The listing builds one solid part. Answer for the finished solid, in the listing's coordinates (mm). A direction names the side the tool comes from. Give positions to 0.01 mm unless a question says otherwise; leave off trailing zeros. Write each loop counter-clockwise with the first axis right and the second up, starting at its lowest first coordinate (ties: lowest second). Pieces come first, ordered by that corner, then holes. Notation, with made-up numbers: (80.5, 17.5) - (86.5, 17.5) arc R19 ccw to (86.5, 48.5) - close; hole circle Ø11 at (54.5, -29). An arc over 180 degrees is marked (long way). Answer as CSV lines item,"result". Start each with the question number.
(1) Each of these flat-tipped pins is pushed along its axis until it touches: pin 1 Ø1.6 at (y, z) = (-13.5, 66.5) entering from -X; pin 2 Ø5 at (x, z) = (3.5, 42) entering from -Y; pin 3 Ø0.6 at (y, z) = (13, 65.5) entering from +X; pin 4 Ø2 at (y, z) = (1, 15) entering from +X. Where does it stop, or does it pass through?
(2) Find section A-A (x = -8). Write down the section's boundary in (y, z), then the cut area to 3 significant figures.
(3) For faces 1 (the face through (-1.5, 0.07, 69.97)), 2 (the face through (-9, -16, 50)), 3 (the face through (-0.524, -13, 66)), 4 (the face through (0.524, -13, 70)), 5 (the face through (0.524, 13, 70)), determine the directions among +Z, -Z, +X, -X, +Y, -Y from which every point of the face is accessible in a straight line to the end or side of a thin tool.
(4) For a pull along Z with two mould halves and no side action, classify faces 6 (the face through (0.524, -13, 66)), 7 (the face through (-9, -16, 10)), 8 (the face through (-18.846, 5.935, 29.72)), 9 (the face through (-16.607, 0, 63)) as pulls with the +Z half, pulls with the -Z half, needs draft (parallel to the pull), parting line crosses it, or undercut.
(5) Find section C-C (z = 30). Write down the section's boundary in (x, y).
(6) Straight lines are drawn through the part: probe 1 along Z at (x, y) = (-14.5, 4); probe 2 along Z at (x, y) = (4.5, 18.5); probe 3 along Z at (x, y) = (9.5, -15). For each, find the intervals that lie inside material, in ascending order.
(7) Find section D-D (y = 13.5). Write down the section's boundary in (x, z).
from build123d import *

# Parameters (mm, degrees)
SKETCH1_R           = 18
BOSS_EXTRUDE1_DEPTH = 65
BOSS_EXTRUDE2_START = -10
SKETCH2_R           = 19.758093793
SKETCH2_R_2         = 18
BOSS_EXTRUDE2_DEPTH = 40
SKETCH3_R           = 1.5
BOSS_EXTRUDE3_DEPTH = 14
SKETCH4_R           = 9
BOSS_EXTRUDE4_DEPTH = 2
SKETCH5_R           = 17
BOSS_EXTRUDE5_DEPTH = 1
BOSS_EXTRUDE6_START = -3
SKETCH6_R           = 9
BOSS_EXTRUDE6_DEPTH = 4
SKETCH7_W           = 4.467838664
SKETCH7_H           = 2.096744874
SKETCH7_W_2         = 4.5697238
CUT_EXTRUDE1_DEPTH  = 5
SKETCH8_W           = 1.048372436
SKETCH8_H           = 4.665257343
BOSS_EXTRUDE7_DEPTH = 7
CHAMFER1_SIZE       = 1


with BuildPart() as part:
    # Sketch1 → Boss-Extrude1 (new body)
    with BuildSketch(Plane.XY):
        Circle(SKETCH1_R)
    extrude(amount=BOSS_EXTRUDE1_DEPTH)

    # Sketch2 → Boss-Extrude2 (add)
    with BuildSketch(Plane(origin=(0, 0, 0), x_dir=(-1, 0, 0), z_dir=(0, 0, -1)).offset(BOSS_EXTRUDE2_START)):
        Circle(SKETCH2_R)
        Circle(SKETCH2_R_2, mode=Mode.SUBTRACT)
    extrude(amount=-BOSS_EXTRUDE2_DEPTH)

    # Sketch3 → Boss-Extrude3 (add)
    with BuildSketch(Plane.XY.offset(65)):
        Circle(SKETCH3_R)
    extrude(amount=BOSS_EXTRUDE3_DEPTH)

    # Sketch4 → Boss-Extrude4 (add)
    with BuildSketch(Plane.XY.offset(65)):
        Circle(SKETCH4_R)
    extrude(amount=BOSS_EXTRUDE4_DEPTH)

    # Sketch5 → Boss-Extrude5 (add)
    with BuildSketch(Plane.XY.offset(67)):
        Circle(SKETCH5_R)
    extrude(amount=BOSS_EXTRUDE5_DEPTH)

    # Sketch6 → Boss-Extrude6 (add)
    with BuildSketch(Plane.XY.offset(79).offset(BOSS_EXTRUDE6_START)):
        Circle(SKETCH6_R)
    extrude(amount=-BOSS_EXTRUDE6_DEPTH)

    # Sketch7 → Cut-Extrude1 (cut)
    with BuildSketch(Plane.XY.offset(65)):
        with Locations((18.943203886, 0)):
            Rectangle(SKETCH7_W, SKETCH7_H)
        with Locations((-18.892261318, 0)):
            Rectangle(SKETCH7_W_2, SKETCH7_H)
    extrude(amount=-CUT_EXTRUDE1_DEPTH, mode=Mode.SUBTRACT)

    # Sketch8 → Boss-Extrude7 (add)
    with BuildSketch(Plane.XY.offset(65)):
        with Locations((0, 13.130864768)):
            Rectangle(SKETCH8_W, SKETCH8_H)
        with Locations((0, -13.130864768)):
            Rectangle(SKETCH8_W, SKETCH8_H)
    extrude(amount=BOSS_EXTRUDE7_DEPTH)

    # Chamfer1
    chamfer1_edges = [part.edges().sort_by_distance(p)[0] for p in [
        (0, -15.463493439, 72),
        (0, -10.798236096, 72),
        (0, 15.463493439, 72),
        (0, 10.798236096, 72),
    ]]
    chamfer(chamfer1_edges, length=CHAMFER1_SIZE)


solid = part.part
Result set:
1,pin 1,"x = -11.1"
1,pin 2,"y = -19.73"
1,pin 3,"x = 0.52"
1,pin 4,"x = 19.76"
2,outline,"(-18.07, 10) - (-16.12, 10) - (-16.12, 0) - (16.12, 0) - (16.12, 10) - (18.07, 10) - (18.07, 50) - (16.12, 50) - (16.12, 65) - (4.12, 65) - (4.12, 67) - (15, 67) - (15, 68) - (-15, 68) - (-15, 67) - (-4.12, 67) - (-4.12, 65) - (-16.12, 65) - (-16.12, 50) - (-18.07, 50) - close; (-4.12, 72) - (4.12, 72) - (4.12, 76) - (-4.12, 76) - close"
2,area,"2,330 mm^2"
3,face 1,"none"
3,face 2,"+Z"
3,face 3,"-X, -Y"
3,face 4,"+Z, +X, -Y"
3,face 5,"+Z, +X, +Y"
4,face 6,"undercut"
4,face 7,"pulls with the -Z half"
4,face 8,"needs draft"
4,face 9,"undercut"
5,outline,"circle Ø39.52 at (0, 0)"
6,probe 1,"0 to 65, 67 to 68"
6,probe 2,"10 to 50"
6,probe 3,"0 to 65"
7,outline,"(-14.43, 10) - (-11.91, 10) - (-11.91, 0) - (11.91, 0) - (11.91, 10) - (14.43, 10) - (14.43, 50) - (11.91, 50) - (11.91, 65) - (0.52, 65) - (0.52, 67) - (10.33, 67) - (10.33, 68) - (0.52, 68) - (0.52, 72) - (-0.52, 72) - (-0.52, 68) - (-10.33, 68) - (-10.33, 67) - (-0.52, 67) - (-0.52, 65) - (-11.91, 65) - (-11.91, 50) - (-14.43, 50) - close"
